Autodesk Inventor part; units mm, degrees
ref_plane "YZ Plane" through (0, 0, 0) normal (1, 0, 0) x (0, 1, 0)
ref_plane "XZ Plane" through (0, 0, 0) normal (0, 1, 0) x (-1, 0, 0)
ref_plane "XY Plane" through (0, 0, 0) normal (0, 0, 1) x (1, 0, 0)
sketch "Sketch1" plane through (0, 0, 0) normal (0, 1, 0) x (-1, 0, 0)
  circle A0 centre (0, 0) radius 3
  circle A1 centre (0, 0) radius 5
  circle A2 centre (0, 0) radius 3.65
  dimension "d0" = 6
  dimension "d1" = 10
  dimension "d2" = 7.3
extrude "Extrusion1" add sketch "Sketch1" along normal blind 4 contours A1
extrude "Extrusion2" add sketch "Sketch1" along normal blind 1.5 from surface at 4 contours A1 | A2
chamfer "Chamfer1" distance 0.5 angle 45 1 edges at (3.65, 0, 0)
properties part number "TransmissionBeltTensionerRoller"
CAD build for the part. Positions are in the model's coordinates, mm. A direction names the side the tool comes from. Round coordinates to 2 decimals unless told otherwise and drop trailing zeros. Loops run counter-clockwise (first coordinate to the right, second up) from the corner with the lowest first, then second, coordinate; pieces in that order, holes last. Notation, with made-up numbers: M 84.25,2.25 L 107.25,2.25 A35 cw 107.25,39.25 Z; hole C -6.5,-13.5 d9. An arc over 180 degrees is marked long. Use a Markdown table: item, result. Add a question column.
(1) Flat gauge pins, fed straight in: pin 1 (2 mm diameter, centred on x = 3, y = 2.5, fed in from +Z); pin 2 (1.5 mm diameter, centred on x = 3, y = 4.5, fed in from -Z); pin 3 (6 mm diameter, centred on x = -0.5, z = -0.5, fed in from -Y). Where does each tip first touch, or does it go through?
(2) Drill centre lines: line 1 (Z direction, x = 0, y = 5.05); line 2 (Z direction, x = -3, y = 2.3); line 3 (Y direction, x = 3, z = -1.5). Where is each one in solid material? Low to high.
(3) Cut at A-A (z = 0). Give the cut face in (x, y).
(4) Which spindle directions (+Z, -Z, +X, -X, +Y, -Y) get a long thin tool onto all of the face, cutting with end or side? Do faces 1 (the face through (2, 0, 4)), 2 (the face through (1, 4, -3)). Say none if no direction does.
(5) Cut at C-C (y = 2.85). Give the cut face in (x, z), and give its area (3 significant figures).
(6) Cut at B-B (x = 0). Give the cut face in (y, z).
Geometry says:
| question | item | result |
|---|---|---|
| 1 | pin 1 | stops at z = 4.58 |
| 1 | pin 2 | stops at z = -4.47 |
| 1 | pin 3 | stops at y = 0.44 |
| 2 | line 1 | z = -5 to -3, 3 to 5 |
| 2 | line 2 | z = -4 to -2.08, 2.08 to 4 |
| 2 | line 3 | y = 4 to 5.5 |
| 3 | outline | M -5,0 L -4.15,0 L -3.65,0.5 L -3.65,4 L -3,4 L -3,5.5 L -5,5.5 Z; M 3,4 L 3.65,4 L 3.65,0.5 L 4.15,0 L 5,0 L 5,5.5 L 3,5.5 Z |
| 4 | face 1 | +Z, -Z, +X, -X, -Y |
| 4 | face 2 | -Y |
| 5 | outline | C 0,0 d10; hole C 0,0 d7.3 |
| 5 | area | 36.7 mm² |
| 6 | outline | M 0,-5 L 5.5,-5 L 5.5,-3 L 4,-3 L 4,-3.65 L 0.5,-3.65 L 0,-4.15 Z; M 0,4.15 L 0.5,3.65 L 4,3.65 L 4,3 L 5.5,3 L 5.5,5 L 0,5 Z |
